```python
from build123d import *

# Parameters (mm, degrees)
SKETCH1_W           = 20
SKETCH1_H           = 20
SKETCH1_W_2         = 16
SKETCH1_H_2         = 16
BOSS_EXTRUDE1_DEPTH = 242
SKETCH2_R           = 3
CUT_EXTRUDE1_DEPTH  = 244.030862238


with BuildPart() as part:
    # Sketch1 → Boss-Extrude1 (new, symmetric)
    with BuildSketch(Plane(origin=(0, 0, 0), x_dir=(0, 0, -1), z_dir=(1, 0, 0))):
        Rectangle(SKETCH1_W, SKETCH1_H)
        Rectangle(SKETCH1_W_2, SKETCH1_H_2, mode=Mode.SUBTRACT)
    extrude(amount=BOSS_EXTRUDE1_DEPTH, both=True)

    # Sketch2 → Cut-Extrude1 (cut, through all)
    with BuildSketch(Plane(origin=(0, 10, 0), x_dir=(1, 0, 0), z_dir=(0, 1, 0))):
        with Locations(Location((212, 0, 0), (0, 0, 270))):
            Circle(SKETCH2_R)
        with Locations(Location((232, 0, 0), (0, 0, 270))):
            Circle(SKETCH2_R)
        with Locations(Location((-232, 0, 0), (0, 0, 270))):
            Circle(SKETCH2_R)
        with Locations(Location((-212, 0, 0), (0, 0, 270))):
            Circle(SKETCH2_R)
    extrude(amount=-CUT_EXTRUDE1_DEPTH, mode=Mode.SUBTRACT)


solid = part.part
```
Verification items for the finished model (mm, model axes). A direction names the side the tool comes from. Coordinates: 2 decimals unless noted, no trailing zeros. Loops run counter-clockwise (first coordinate to the right, second up) from the corner with the lowest first, then second, coordinate; pieces in that order, holes last. Notation, with made-up numbers: (-3.5, 88) - (24.5, 88) arc R23 ccw to (24.5, 112) - close; hole circle Ø8 at (20, -23). An arc over 180 degrees is marked (long way). Put each result on its own line as item: value.
Item 1: Section check B-B (x = -177.5). Enter the section's corners in (y, z).
Conclusion:
outline: (-10, -10) - (10, -10) - (10, 10) - (-10, 10) - close; hole (-8, -8) - (8, -8) - (8, 8) - (-8, 8) - close
Item 2: Section check A-A (y = 0.5). Enter the section's corners in (x, z).
Conclusion:
outline: (-242, -10) - (242, -10) - (242, -8) - (-242, -8) - close; (-242, 8) - (242, 8) - (242, 10) - (-242, 10) - close
Item 3: Scan lines: line 1 along X through (y, z) = (-9.1, 0); line 2 along Z through (x, y) = (117, 3.5). Record each from-to range of solid material in increasing order.
Conclusion:
line 1: x = -242 to -235, -229 to -215, -209 to 209, 215 to 229, 235 to 242
line 2: z = -10 to -8, 8 to 10
Item 4: Draft check along Y on faces 3 (the face through (3, -10, 0)), 4 (the face through (3, 0, -10)), 5 (the face through (3, 0, -8)). Enter one of: pulls with the +Y half, pulls with the -Y half, needs draft (parallel to the pull), parting line crosses it, or undercut.
Conclusion:
face 3: pulls with the -Y half
face 4: needs draft
face 5: undercut
Item 5: Set-up check for faces 1 (the face through (-242, 0, 9)), 2 (the face through (3, 0, 8)): record each of +Z, -Z, +X, -X, +Y, -Y from which the full face is reachable in a straight line by a thin tool's end or side.
Conclusion:
face 1: +Z, -Z, -X, +Y, -Y
face 2: +X, -X
Item 6: Gauge pin test, flat end, axial feed: pin 1 Ø5 at (x, z) = (-212, 0) entering from +Y. Record the tip position at first contact, or that the pin passes through.
Conclusion:
pin 1: passes through
Item 7: Section check C-C (z = 0). Give the number of separate pieces and of enclosed holes in the cut face, then the cut area to 3 significant figures.
Conclusion:
separate pieces: 10
enclosed holes: 0
area: 1,840 mm2
